Here's how the part is built. I have some questions about the finished solid (model axes, mm). Coordinates: 2 decimals unless noted, no trailing zeros. Loops run counter-clockwise (first coordinate to the right, second up) from the corner with the lowest first, then second, coordinate; pieces in that order, holes last. Notation, with made-up numbers: (-29.75, 47.25) - (4.25, 47.25) arc R24 ccw to (4.25, 71.25) - close; hole circle Ø9 at (27, 15.25). An arc over 180 degrees is marked (long way). Use a Markdown table: item, result.
```python
from build123d import *

# Parameters (mm, degrees)
ESQUISSE1_W             = 32
ESQUISSE1_H             = 24
BOSS_EXTRU_1_DEPTH      = 8
ESQUISSE2_R             = 2
ENL_V_MAT_EXTRU_1_DEPTH = 8
ENL_V_MAT_EXTRU_2_REACH = 37.543
ESQUISSE3_R             = 1.65
ENL_V_MAT_EXTRU_3_REACH = 37.543
ESQUISSE4_R             = 1.65


with BuildPart() as part:
    # Esquisse1 → Boss.-Extru.1 (new body)
    with BuildSketch(Plane(origin=(0, 0, 0), x_dir=(1, 0, 0), z_dir=(0, 1, 0))):
        with Locations((3.126436782, 1.24137931)):
            Rectangle(ESQUISSE1_W, ESQUISSE1_H)
    extrude(amount=BOSS_EXTRU_1_DEPTH)

    # Esquisse2 → Enlèv. mat.-Extru.1 (cut)
    with BuildSketch(Plane(origin=(0, 8, 0), x_dir=(1, 0, 0), z_dir=(0, 1, 0))):
        with Locations(Location((3.126436782, 1.24137931, 0), (0, 0, 270))):
            Circle(ESQUISSE2_R)
    extrude(amount=-ENL_V_MAT_EXTRU_1_DEPTH, mode=Mode.SUBTRACT)

    # Esquisse3 → Enlèv. mat.-Extru.2 (cut, up to next)
    with BuildSketch(Plane.ZY.offset(12.873563218), mode=Mode.PRIVATE) as enl_v_mat_extru_2_sk1:
        with Locations((-9.24137931, 4)):
            Circle(ESQUISSE3_R)
    enl_v_mat_extru_2_tool1 = extrude(enl_v_mat_extru_2_sk1.sketch, amount=-ENL_V_MAT_EXTRU_2_REACH, mode=Mode.PRIVATE) & part.part
    add(enl_v_mat_extru_2_tool1.solids().sort_by_distance((-12.873563, 4, -9.241379))[0], mode=Mode.SUBTRACT)

    # Esquisse4 → Enlèv. mat.-Extru.3 (cut, up to next)
    with BuildSketch(Plane.ZY.offset(12.873563218), mode=Mode.PRIVATE) as enl_v_mat_extru_3_sk1:
        with Locations((6.75862069, 4)):
            Circle(ESQUISSE4_R)
    enl_v_mat_extru_3_tool1 = extrude(enl_v_mat_extru_3_sk1.sketch, amount=-ENL_V_MAT_EXTRU_3_REACH, mode=Mode.PRIVATE) & part.part
    add(enl_v_mat_extru_3_tool1.solids().sort_by_distance((-12.873563, 4, 6.758621))[0], mode=Mode.SUBTRACT)


solid = part.part
```
Q1. I want a section at B-B, the plane z = -10.5. Write out the boundary of the cut face in (x, y), then the cut area to 3 significant figures.
Check values:
| item | result |
|---|---|
| outline | (-12.87, 0) - (19.13, 0) - (19.13, 2.93) - (-12.87, 2.93) - close; (-12.87, 5.07) - (19.13, 5.07) - (19.13, 8) - (-12.87, 8) - close |
| area | 188 mm^2 |
Q2. Please list where these lines run through material, in increasing order: L1, parallel to Z at x = -4.5, y = 5.5; L2, parallel to Z at x = 3, y = 1.75; L3, parallel to Z at x = -0.5, y = 4.25. Write a range as from..to.
Check values:
| item | result |
|---|---|
| L1 | -13.24..-9.93, -8.55..6.07, 7.45..10.76 |
| L2 | -13.24..-3.24, 0.75..10.76 |
| L3 | -13.24..-10.87, -7.61..5.13, 8.39..10.76 |
Q3. I want a section at C-C, the plane x = 13. Write out the boundary of the cut face in (y, z).
Check values:
| item | result |
|---|---|
| outline | (0, -13.24) - (8, -13.24) - (8, 10.76) - (0, 10.76) - close; hole circle Ø3.3 at (4, -9.24); hole circle Ø3.3 at (4, 6.76) |
Q4. I want a section at A-A, the plane y = 4. Write out the boundary of the cut face in (x, z), then the cut area to 3 significant figures.
Check values:
| item | result |
|---|---|
| outline | (-12.87, -13.24) - (19.13, -13.24) - (19.13, -10.89) - (-12.87, -10.89) - close; (-12.87, -7.59) - (19.13, -7.59) - (19.13, 5.11) - (-12.87, 5.11) - close; (-12.87, 8.41) - (19.13, 8.41) - (19.13, 10.76) - (-12.87, 10.76) - close; hole circle Ø4 at (3.13, -1.24) |
| area | 544 mm^2 |
Q5. Will this pin go through, and if not, where does the flat tip stop? P1, Ø3, axis at y = 4, z = 6.76, coming from the +X side.
Check values:
| item | result |
|---|---|
| P1 | through |
Q6. I want a section at D-D, the plane y = 1.75. Write out the boundary of the cut face in (x, z), then the cut area to 3 significant figures.
Check values:
| item | result |
|---|---|
| outline | (-12.87, -13.24) - (19.13, -13.24) - (19.13, 10.76) - (-12.87, 10.76) - close; hole circle Ø4 at (3.13, -1.24) |
| area | 755 mm^2 |
Q7. If we mould it in two halves opening along Z, with no side actions, what happens to faces 1 (the face through (3, 4, -13.241)), 2 (the face through (2.902, 3.368, -7.717)), 3 (the face through (3, 8, -4))? For each: pulls with the +Z half, pulls with the -Z half, needs draft (parallel to the pull), parting line crosses it, or undercut.
Check values:
| item | result |
|---|---|
| face 1 | pulls with the -Z half |
| face 2 | undercut |
| face 3 | needs draft |
